For this review, take the finished solid that the model builds, in its own axes (mm). Face numbers are marked on the shaded views. A direction names the side the tool comes from. Round coordinates to 2 decimals unless told otherwise and drop trailing zeros. Order: outer loops, then holes, each group sorted by start corner. A loop starts at its lowest first (then second) coordinate and runs counter-clockwise, first axis right, second up. Notation, with made-up numbers: (1, -28) -> (42, -28) arc R25 ccw to (42, -9) -> close; hole circle Ø2 at (50, 26). An arc over 180 degrees is marked (long way). Use a Markdown table: item, result. Add a question column.
1) Draft analysis for pull direction Z (two halves, no side actions). For the marked faces 4, 5 and 6, state which applies: pulls with the +Z half, pulls with the -Z half, needs draft (parallel to the pull), parting line crosses it, or undercut.
2) Consider section D-D (x = -8). State the section outline as (y, z) points.
3) Consider section C-C (z = 0). State the section outline as (x, y) points.
4) Machinability: for the marked faces 1, 2 and 3, which of the approach directions +Z, -Z, +X, -X, +Y, -Y give a long, thin tool a straight path to every point of the face, cutting with its end or side? Answer none if there is none.
5) Clearance check with flat-ended pins moving along their axes: P1, Ø3.5, axis at x = 14, z = -10, coming from the +Y side; P2, Ø0.5, axis at x = -17, z = 0.5, coming from the +Y side; P3, Ø5, axis at x = 13.5, z = 0, coming from the +Y side. State where each tip first meets the part, or that it passes through.
6) Consider section A-A (y = 3.5). State the section outline as (x, z) points.
7) Wall thickness on line 1 along X through (y, z) = (4.25, 7.25); line 2 along X through (y, z) = (5.25, -9.5); line 3 along X through (y, z) = (5.75, 4.25): over which ranges is each line inside the solid? List them lowest first. Write a range as [from, to].
8) Consider section B-B (z = -10.75). State the section outline as (x, y) points, plus the area to 3 significant figures.
```python
from build123d import *

# Parameters (mm, degrees)
SKETCH1_W           = 35.7
SKETCH1_H           = 28.2
BOSS_EXTRUDE1_DEPTH = 7
SKETCH2_W           = 34.4
SKETCH2_H           = 25.8
CUT_EXTRUDE1_DEPTH  = 1.5
CUT_EXTRUDE2_DEPTH  = 4.5
SKETCH4_W           = 22.4
SKETCH4_H           = 1.2
CUT_EXTRUDE3_DEPTH  = 6
SKETCH5_W           = 1
SKETCH5_H           = 6
BOSS_EXTRUDE2_DEPTH = 1
SKETCH6_W           = 6
SKETCH6_H           = 2.2
BOSS_EXTRUDE3_DEPTH = 1.5


with BuildPart() as part:
    # Sketch1 → Boss-Extrude1 (new body)
    with BuildSketch(Plane(origin=(0, 0, 0), x_dir=(1, 0, 0), z_dir=(0, 1, 0))):
        Rectangle(SKETCH1_W, SKETCH1_H)
    extrude(amount=BOSS_EXTRUDE1_DEPTH)

    # Sketch2 → Cut-Extrude1 (cut)
    with BuildSketch(Plane(origin=(0, 7, 0), x_dir=(1, 0, 0), z_dir=(0, 1, 0))):
        with Locations((-0.65, 0)):
            Rectangle(SKETCH2_W, SKETCH2_H)
    extrude(amount=-CUT_EXTRUDE1_DEPTH, mode=Mode.SUBTRACT)

    # Sketch3 → Cut-Extrude2 (cut)
    with BuildSketch(Plane(origin=(0, 5.5, 0), x_dir=(1, 0, 0), z_dir=(0, 1, 0))):
        Polygon((-10.85, 12.9), (-10.85, -12.9), (11.55, -12.9), (11.55, -8.4), (16.55, -8.4), (16.55, 8.4), (11.55, 8.4), (11.55, 12.9), align=None)
    extrude(amount=-CUT_EXTRUDE2_DEPTH, mode=Mode.SUBTRACT)

    # Sketch4 → Cut-Extrude3 (cut)
    with BuildSketch(Plane(origin=(0, 7, 0), x_dir=(1, 0, 0), z_dir=(0, 1, 0))):
        with Locations((0.35, -13.5)):
            Rectangle(SKETCH4_W, SKETCH4_H)
    cut_extrude3 = extrude(amount=-CUT_EXTRUDE3_DEPTH, mode=Mode.SUBTRACT)

    # Mirror1: Cut-Extrude3 across plane
    add(cut_extrude3.mirror(Plane.XY), mode=Mode.SUBTRACT)

    # Sketch5 → Boss-Extrude2 (add)
    with BuildSketch(Plane(origin=(0, 5.5, 0), x_dir=(1, 0, 0), z_dir=(0, 1, 0))):
        with Locations((-17.35, 0)):
            Rectangle(SKETCH5_W, SKETCH5_H)
    extrude(amount=BOSS_EXTRUDE2_DEPTH)

    # Sketch6 → Boss-Extrude3 (add)
    with BuildSketch(Plane(origin=(0, 5.5, 0), x_dir=(1, 0, 0), z_dir=(0, 1, 0))):
        with Locations((-14.85, -11.8)):
            Rectangle(SKETCH6_W, SKETCH6_H)
    extrude(amount=BOSS_EXTRUDE3_DEPTH)


solid = part.part
```
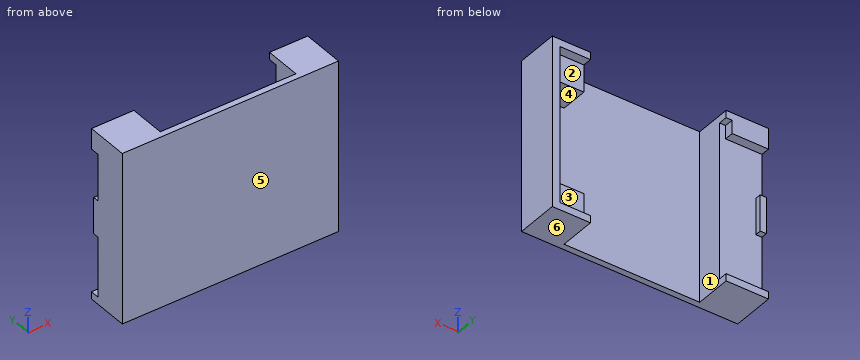
Results list:
| question | item | result |
|---|---|---|
| 1 | face 4 | undercut |
| 1 | face 5 | needs draft |
| 1 | face 6 | pulls with the -Z half |
| 2 | outline | (0, -14.1) -> (1, -14.1) -> (1, 14.1) -> (0, 14.1) -> close |
| 3 | outline | (-17.85, 0) -> (17.85, 0) -> (17.85, 7) -> (16.55, 7) -> (16.55, 1) -> (-10.85, 1) -> (-10.85, 5.5) -> (-16.85, 5.5) -> (-16.85, 6.5) -> (-17.85, 6.5) -> close |
| 4 | face 1 | +Z, -Z, +Y |
| 4 | face 2 | +Y |
| 4 | face 3 | -X, +Y |
| 5 | P1 | y = 5.5 |
| 5 | P2 | y = 6.5 |
| 5 | P3 | y = 1 |
| 6 | outline | (-17.85, -14.1) -> (-10.85, -14.1) -> (-10.85, 14.1) -> (-17.85, 14.1) -> close; (11.55, -14.1) -> (17.85, -14.1) -> (17.85, 14.1) -> (11.55, 14.1) -> (11.55, 8.4) -> (16.55, 8.4) -> (16.55, -8.4) -> (11.55, -8.4) -> close |
| 7 | line 1 | [-17.85, -10.85], [16.55, 17.85] |
| 7 | line 2 | [-17.85, -10.85], [11.55, 17.85] |
| 7 | line 3 | [16.55, 17.85] |
| 8 | outline | (-17.85, 0) -> (17.85, 0) -> (17.85, 7) -> (16.55, 7) -> (16.55, 5.5) -> (11.55, 5.5) -> (11.55, 1) -> (-10.85, 1) -> (-10.85, 5.5) -> (-17.85, 5.5) -> close |
| 8 | area | 97.5 mm2 |
